from build123d import *

# Parameters (mm, degrees)
SKETCH_1_R      = 5
EXTRUDE_1_DEPTH = 25
SKETCH_2_R      = 4
SKETCH_4_R      = 10
EXTRUDE_2_DEPTH = 7


with BuildPart() as part:
    # ｽｹｯﾁ1 → ﾎﾞｽ - 押し出し1 (new body)
    with BuildSketch(Plane.XY):
        Circle(SKETCH_1_R)
    extrude(amount=EXTRUDE_1_DEPTH)

    # ｽｲｰﾌﾟ1: sweep along a path in ｽｹｯﾁ3
    with BuildLine(Plane(origin=(0, 0, 0), x_dir=(0, 0, -1), z_dir=(1, 0, 0))) as sweep_1_path:
        CenterArc((-41.5, 0), 16.5, 0, 360)
    # ｽｹｯﾁ2 → ｽｲｰﾌﾟ1 (sweep)
    with BuildSketch(Plane(origin=(0, 0, 0), x_dir=(1, 0, 0), z_dir=(0, 1, 0))):
        with Locations((0, -25)):
            Circle(SKETCH_2_R)
    sweep(path=sweep_1_path.line)

    # ｽｹｯﾁ4 → ﾎﾞｽ - 押し出し2 (add)
    with BuildSketch(Plane(origin=(0, 0, 18), x_dir=(-1, 0, 0), z_dir=(0, 0, -1))):
        Circle(SKETCH_4_R)
    extrude(amount=-EXTRUDE_2_DEPTH)


solid = part.part
The listing builds one solid part. Answer for the finished solid, in the listing's coordinates (mm). A direction names the side the tool comes from. Round coordinates to 2 decimals unless told otherwise and drop trailing zeros. Order: outer loops, then holes, each group sorted by start corner. A loop starts at its lowest first (then second) coordinate and runs counter-clockwise, first axis right, second up. Notation, with made-up numbers: M 43,37.5 L 75,37.5 A29 cw 75,58.5 Z; hole C 60,71 d10. An arc over 180 degrees is marked long. Answer in a Markdown table with one row per item. Add a question column.
1) Which of the six approach directions +Z, -Z, +X, -X, +Y, -Y give full straight-line access (tool end or side, diameter ignored) to faces 1 (the face through (-9.54, 3, 21.45)), 2 (the face through (0, 0, 0))?
2) The part is cut by section A-A on x = 0. Determine the outline of the cut face in (y, z).
3) The part is cut by section B-B on x = 6. Determine the outline of the cut face in (y, z), plus the area to 3 significant figures.
4) Flat-ended cylindrical pins translate along their axes: pin 1 Ø4 at (x, y) = (-3.5, 6) entering from +Z; pin 2 Ø1 at (x, z) = (4.5, 20) entering from -Y; pin 3 Ø10 at (x, y) = (-3, -13) entering from +Z; pin 4 Ø1.5 at (x, z) = (-5, 34) entering from -Y. Find the tip coordinate at first contact, or state that the pin passes through.
5) Consider line 1 along Z through (x, y) = (-4.25, -4); line 2 along Z through (x, y) = (1.75, -10); line 3 along Z through (x, y) = (2.25, -10.5). Determine where each line is inside the solid, lowest interval first. Write a range as from..to.
6) The part is cut by section C-C on x = -7.25. Determine the outline of the cut face in (y, z).
Findings below:
| question | item | result |
|---|---|---|
| 1 | face 1 | -Z |
| 1 | face 2 | -Z, +X, -X, +Y, -Y |
| 2 | outline | M -10,18 L -5,18 L -5,0 L 5,0 L 5,18 L 10,18 L 10,23.6 A20.5 ccw long -10,23.6 Z; hole C 0,41.5 d25 |
| 3 | outline | M -8,18 L 8,18 L 8,25 L -8,25 Z |
| 3 | area | 112 mm² |
| 4 | pin 1 | stops at z = 60.96 |
| 4 | pin 2 | stops at y = -9.17 |
| 4 | pin 3 | stops at z = 60.06 |
| 4 | pin 4 | passes through |
| 5 | line 1 | z = 18..25 |
| 5 | line 2 | z = 24.07..33.35, 49.65..58.93 |
| 5 | line 3 | z = 24.7..33.51, 49.49..58.3 |
| 6 | outline | M -6.89,18 L 6.89,18 L 6.89,25 L -6.89,25 Z |
